Can you work these out from the model? Positions are in its coordinate system, mm. A direction names the side the tool comes from. Coordinates: 2 decimals unless noted, no trailing zeros. Loops run counter-clockwise (first coordinate to the right, second up) from the corner with the lowest first, then second, coordinate; pieces in that order, holes last. Notation, with made-up numbers: M 42,11 L 46,11 A16 cw 46,37 Z; hole C 39,-31.5 d4. An arc over 180 degrees is marked long. Answer as a JSON object with one key per item and string values. Group by question number.
Item 1: Suppose I cut it at A-A (z = 279.4). Write out the boundary of the cut face in (x, y) (3 decimals), then the cut area to 3 significant figures.
Item 2: Suppose I cut it at C-C (z = 767). Write out the boundary of the cut face in (x, y) (3 decimals).
Item 3: Which directions (+Z, -Z, +X, -X, +Y, -Y) give clear straight access to the entire face, cutting with the end or side of a thin tool? Please do faces 1 (the flat face through (16, 3.175, 413)), 2 (the cylindrical face through (1.61, 38.426, 537.601)).
Item 4: Suppose I cut it at B-B (x = 21). Write out the boundary of the cut face in (y, z) (3 decimals), then the cut area to 3 significant figures.
Item 5: If I drill on line 1 (Y direction, x = 30.3, z = 698.5) (3 decimals); line 2 (X direction, y = 19, z = 320.5) (3 decimals); line 3 (Y direction, x = 18, z = 38) (3 decimals), over which ranges is the centre line in solid material (lowest first)?
Item 6: We'd pull the mould along Z, two halves only. Please class faces 3 (the flat face through (16, 0, 413)), 4 (the cylindrical face through (1.61, 46.77, 365.63)), 5 (the flat face through (3, 34, 0)): +Z half, -Z half, draft (parallel to the pull), parting line (faces both ways), or undercut.
Item 7: Suppose I cut it at D-D (y = 31.75). Count the separate pieces of the cut face and the enclosed holes in it, then the cut area to 3 significant figures.
```python
from build123d import *

# Parameters (mm, degrees)
SKETCH1_W           = 31.75
SKETCH1_H           = 63.5
SKETCH1_W_2         = 25.4
SKETCH1_H_2         = 57.15
BOSS_EXTRUDE1_DEPTH = 838.2
SKETCH2_R           = 22.225
CUT_EXTRUDE1_DEPTH  = 31.75


with BuildPart() as part:
    # Sketch1 → Boss-Extrude1 (new body)
    with BuildSketch(Plane.XY):
        with Locations((15.875, 31.75)):
            Rectangle(SKETCH1_W, SKETCH1_H)
        with Locations((15.875, 31.75)):
            Rectangle(SKETCH1_W_2, SKETCH1_H_2, mode=Mode.SUBTRACT)
    extrude(amount=BOSS_EXTRUDE1_DEPTH)

    # Sketch2 → Cut-Extrude1 (cut)
    with BuildSketch(Plane(origin=(31.75, 0, 0), x_dir=(0, 0, -1), z_dir=(1, 0, 0))):
        with Locations((-698.5, 31.75)):
            Circle(SKETCH2_R)
        with Locations((-628.65, 31.75)):
            Circle(SKETCH2_R)
        with Locations((-558.8, 31.75)):
            Circle(SKETCH2_R)
        with Locations((-488.95, 31.75)):
            Circle(SKETCH2_R)
        with Locations((-419.1, 31.75)):
            Circle(SKETCH2_R)
        with Locations((-349.25, 31.75)):
            Circle(SKETCH2_R)
        with Locations((-279.4, 31.75)):
            Circle(SKETCH2_R)
        with Locations((-209.55, 31.75)):
            Circle(SKETCH2_R)
        with Locations((-139.7, 31.75)):
            Circle(SKETCH2_R)
    extrude(amount=-CUT_EXTRUDE1_DEPTH, mode=Mode.SUBTRACT)


solid = part.part
```
From the geometry:
{
 "1": {"outline": "M 0,0 L 31.75,0 L 31.75,9.525 L 28.575,9.525 L 28.575,3.175 L 3.175,3.175 L 3.175,9.525 L 0,9.525 Z; M 0,53.975 L 3.175,53.975 L 3.175,60.325 L 28.575,60.325 L 28.575,53.975 L 31.75,53.975 L 31.75,63.5 L 0,63.5 Z", "area": "282 mm2"},
 "2": {"outline": "M 0,0 L 31.75,0 L 31.75,63.5 L 0,63.5 Z; hole M 3.175,3.175 L 28.575,3.175 L 28.575,60.325 L 3.175,60.325 Z"},
 "3": {"face 1": "+Z, -Z", "face 2": "+X, -X"},
 "4": {"outline": "M 0,0 L 3.175,0 L 3.175,838.2 L 0,838.2 Z; M 60.325,0 L 63.5,0 L 63.5,838.2 L 60.325,838.2 Z", "area": "5,320 mm2"},
 "5": {"line 1": "0 to 9.525, 53.975 to 63.5", "line 2": "0 to 3.175, 28.575 to 31.75", "line 3": "0 to 3.175, 60.325 to 63.5"},
 "6": {"face 3": "draft", "face 4": "undercut", "face 5": "-Z half"},
 "7": {"separate pieces": "20", "enclosed holes": "0", "area": "2,780 mm2"}
}
